Can you work these out from the drawing? Everything is in mm from the part's minimum corner. Round coordinates to 2 decimals unless told otherwise and drop trailing zeros. Loops run counter-clockwise (first coordinate to the right, second up) from the corner with the lowest first, then second, coordinate; pieces in that order, holes last. Notation, with made-up numbers: (-37.75, 49.25) -> (-13.75, 49.25) arc R14 cw to (-13.75, 71.25) -> close; hole circle Ø6 at (-1, 89). An arc over 180 degrees is marked (long way). One line per item, written item: value.
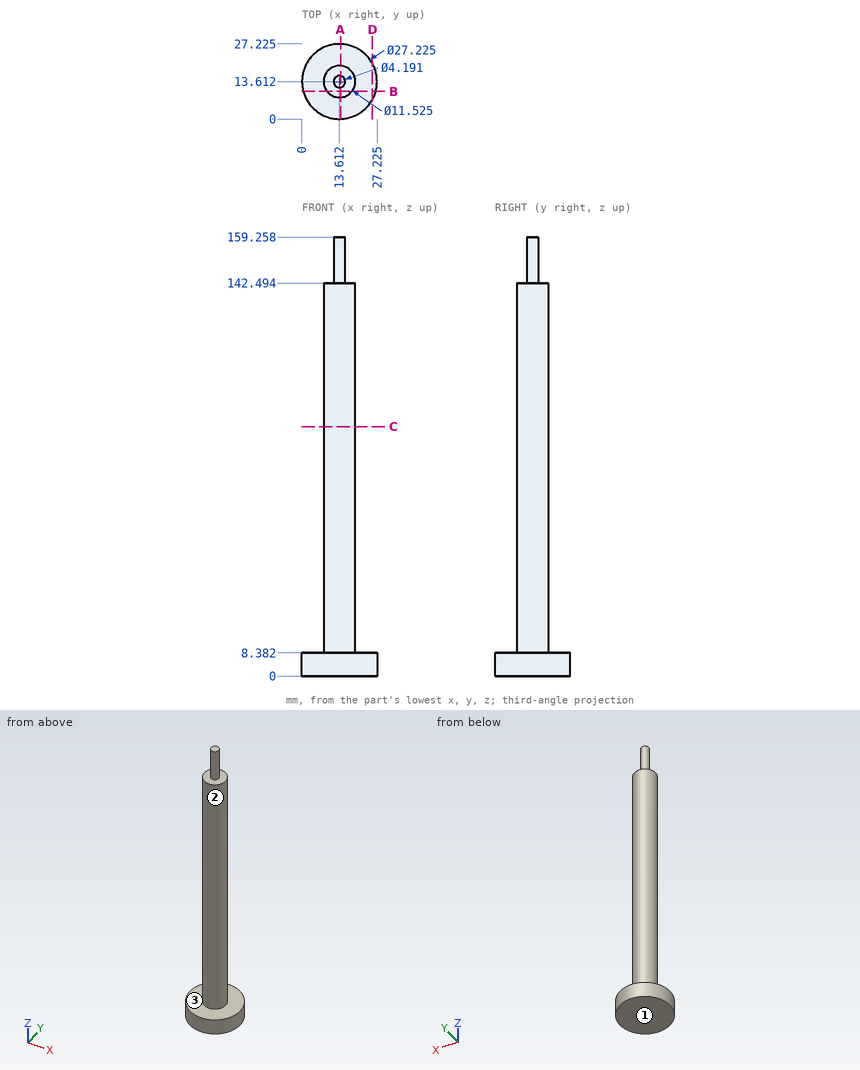
(1) We'd pull the mould along Z, two halves only. Please class the marked faces 1, 2 and 3: +Z half, -Z half, draft (parallel to the pull), parting line (faces both ways), or undercut.
Results below:
face 1: -Z half
face 2: draft
face 3: +Z half
(2) Imagine slicing it at C-C on z = 90.5. Write out the boundary of the cut face in (x, y) (1 decimal), then the cut area to 3 significant figures.
Results below:
outline: circle Ø11.5 at (13.6, 13.6)
area: 104 mm²
(3) Imagine slicing it at D-D on x = 25.5. Write out the boundary of the cut face in (y, z).
Results below:
outline: (6.98, 0) -> (20.24, 0) -> (20.24, 8.38) -> (6.98, 8.38) -> close
(4) Imagine slicing it at A-A on x = 14. Write out the boundary of the cut face in (y, z) (1 decimal), then the cut area to 3 significant figures.
Results below:
outline: (0, 0) -> (27.2, 0) -> (27.2, 8.4) -> (19.4, 8.4) -> (19.4, 142.5) -> (15.7, 142.5) -> (15.7, 159.3) -> (11.6, 159.3) -> (11.6, 142.5) -> (7.9, 142.5) -> (7.9, 8.4) -> (0, 8.4) -> close
area: 1,840 mm²
(5) Imagine slicing it at B-B on y = 10. Write out the boundary of the cut face in (x, z), then the cut area to 3 significant figures.
Results below:
outline: (0.49, 0) -> (26.74, 0) -> (26.74, 8.38) -> (18.1, 8.38) -> (18.1, 142.49) -> (9.12, 142.49) -> (9.12, 8.38) -> (0.49, 8.38) -> close
area: 1,420 mm²
(6) For pin 1 Ø12 at (x, y) = (7, 23) entering from +Z; pin 2 Ø8 at (x, z) = (12, 117.5) entering from +Y (3 decimals); pin 3 Ø10 at (x, y) = (3.5, 9.5) entering from +Z, each with a flat end and sliding along its axis, tell me the tip position at first contact or that it passes through.
Results below:
pin 1: stops at z = 142.49
pin 2: stops at y = 19.375
pin 3: stops at z = 8.38
(7) Please list where these lines run through material, in increasing order: L1, parallel to Z at x = 9.75, y = 4.5; L2, parallel to Y at x = 13.75, z = 94; L3, parallel to Z at x = 12, y = 10.25.
Results below:
L1: z = 0 to 8.38
L2: y = 7.85 to 19.37
L3: z = 0 to 142.49
